from build123d import *

# Parameters (mm, degrees)
SKETCH1_R           = 4
BOSS_EXTRUDE1_DEPTH = 2
SKETCH2_R           = 2.5
BOSS_EXTRUDE2_DEPTH = 40
SKETCH3_OUTSIDE_W   = 18.7
SKETCH3_OUTSIDE_H   = 18.7
CUT_EXTRUDE1_DEPTH  = 10


with BuildPart() as part:
    # Sketch1 → Boss-Extrude1 (new body)
    with BuildSketch(Plane(origin=(0, 0, 0), x_dir=(1, 0, 0), z_dir=(0, 1, 0))):
        Circle(SKETCH1_R)
    extrude(amount=BOSS_EXTRUDE1_DEPTH)

    # Sketch2 → Boss-Extrude2 (add)
    with BuildSketch(Plane(origin=(0, 2, 0), x_dir=(1, 0, 0), z_dir=(0, 1, 0))):
        Circle(SKETCH2_R)
    extrude(amount=BOSS_EXTRUDE2_DEPTH)

    # Sketch3 outside → Cut-Extrude1 (cut)
    with BuildSketch(Plane(origin=(0, 0, 0), x_dir=(-1, 0, 0), z_dir=(0, -1, 0))):
        Rectangle(SKETCH3_OUTSIDE_W, SKETCH3_OUTSIDE_H)
        Polygon((0, 4), (3.464101615, 2), (3.464101615, -2), (0, -4), (-3.464101615, -2), (-3.464101615, 2), align=None, mode=Mode.SUBTRACT)
    extrude(amount=-CUT_EXTRUDE1_DEPTH, mode=Mode.SUBTRACT)


solid = part.part
The listing builds one solid part. Answer for the finished solid, in the listing's coordinates (mm). A direction names the side the tool comes from. Coordinates: 2 decimals unless noted, no trailing zeros. Write each loop counter-clockwise with the first axis right and the second up, starting at its lowest first coordinate (ties: lowest second). Pieces come first, ordered by that corner, then holes. Notation, with made-up numbers: M 78.25,10.5 L 133.25,10.5 A17 cw 133.25,32.5 Z; hole C 38,84 d6. An arc over 180 degrees is marked long. Write each question's results on one line, items separated by ' | '.
Item 1: The part is cut by section D-D on z = 3.5. Determine the outline of the cut face in (x, y), and give its area (3 significant figures).
Answer below:
outline: M -0.87,0 L 0.87,0 L 0.87,2 L -0.87,2 Z | area: 3.46 mm2
Item 2: The part is cut by section C-C on x = -1. Determine the outline of the cut face in (y, z).
Answer below:
outline: M 0,-3.42 L 2,-3.42 L 2,-2.29 L 42,-2.29 L 42,2.29 L 2,2.29 L 2,3.42 L 0,3.42 Z
Item 3: Which of the six approach directions +Z, -Z, +X, -X, +Y, -Y give full straight-line access (tool end or side, diameter ignored) to faces 1 (the face through (0, 2, 3)), 2 (the face through (3.464, 1, 0))?
Answer below:
face 1: +Y | face 2: +Z, -Z, +X, +Y, -Y
Item 4: Consider probe 1 along Z at (x, y) = (0, 7); probe 2 along Z at (x, y) = (2, 25); probe 3 along Y at (x, z) = (0.5, -3.25). Determine where each line is inside the solid, lowest interval first. Write a range as [from, to].
Answer below:
probe 1: [-2.5, 2.5] | probe 2: [-1.5, 1.5] | probe 3: [0, 2]
Item 5: The part is cut by section A-A on z = 1.5. Determine the outline of the cut face in (x, y).
Answer below:
outline: M -3.46,0 L 3.46,0 L 3.46,2 L 2,2 L 2,42 L -2,42 L -2,2 L -3.46,2 Z
Item 6: The part is cut by section B-B on y = 14. Determine the outline of the cut face in (x, z).
Answer below:
outline: C 0,0 d5
Item 7: Given P1, Ø4, axis at y = 6.5, z = -1, coming from the +X side; P2, Ø4, axis at y = 26, z = 0.5, coming from the -X side, each flat-ended and moving along its own axis, determine where each tip first touches the part or whether it passes through.
Answer below:
P1: x = 2.5 | P2: x = -2.5
